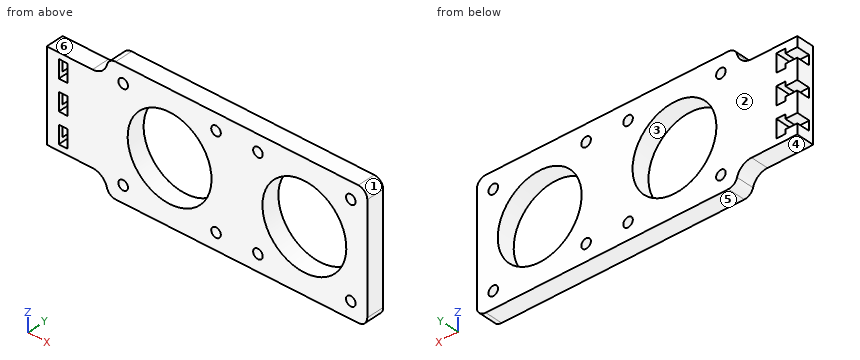
```python
from build123d import *

# Parameters (mm, degrees)
SKETCH_1_W          = 20
SKETCH_1_H          = 30
EXTRUDE_1_DEPTH     = 6
SKETCH_2_W          = 4
SKETCH_2_H          = 3.2
CUT_EXTRUDE_1_DEPTH = 4.5
SKETCH_3_W          = 3
SKETCH_3_H          = 6
CUT_EXTRUDE_2_DEPTH = 14.5
SKETCH_4_W          = 87
SKETCH_4_H          = 42
SKETCH_4_R          = 1.6
SKETCH_4_R_2        = 14
EXTRUDE_2_DEPTH     = 6
FILLET_1_R          = 3
FILLET_2_R          = 5


with BuildPart() as part:
    # 草图1 → 凸台-拉伸1 (new body)
    with BuildSketch(Plane(origin=(0, 0, 0), x_dir=(1, 0, 0), z_dir=(0, 1, 0))):
        with Locations((10, 15)):
            Rectangle(SKETCH_1_W, SKETCH_1_H)
    extrude(amount=EXTRUDE_1_DEPTH)

    # 草图2 → 切除-拉伸1 (cut)
    with BuildSketch(Plane(origin=(0, 6, 0), x_dir=(1, 0, 0), z_dir=(0, 1, 0))):
        with Locations((2, 5)):
            Rectangle(SKETCH_2_W, SKETCH_2_H)
        with Locations((2, 15)):
            Rectangle(SKETCH_2_W, SKETCH_2_H)
        with Locations((2, 25)):
            Rectangle(SKETCH_2_W, SKETCH_2_H)
    extrude(amount=-CUT_EXTRUDE_1_DEPTH, mode=Mode.SUBTRACT)

    # 草图3 → 切除-拉伸2 (cut)
    with BuildSketch(Plane(origin=(0, 6, 0), x_dir=(1, 0, 0), z_dir=(0, 1, 0))):
        with Locations((5.5, 5)):
            Rectangle(SKETCH_3_W, SKETCH_3_H)
        with Locations((5.5, 15)):
            Rectangle(SKETCH_3_W, SKETCH_3_H)
        with Locations((5.5, 25)):
            Rectangle(SKETCH_3_W, SKETCH_3_H)
    extrude(amount=-CUT_EXTRUDE_2_DEPTH, mode=Mode.SUBTRACT)

    # 草图4 → 凸台-拉伸2 (add)
    with BuildSketch(Plane.XZ):
        with Locations((63.5, -15)):
            Rectangle(SKETCH_4_W, SKETCH_4_H)
        with Locations(Location((25.5, 0.5, 0), (0, 0, 270))):
            Circle(SKETCH_4_R, mode=Mode.SUBTRACT)
        with Locations(Location((25.5, -30.5, 0), (0, 0, 90))):
            Circle(SKETCH_4_R, mode=Mode.SUBTRACT)
        with Locations(Location((56.5, -30.5, 0), (0, 0, 90))):
            Circle(SKETCH_4_R, mode=Mode.SUBTRACT)
        with Locations(Location((56.5, 0.5, 0), (0, 0, 270))):
            Circle(SKETCH_4_R, mode=Mode.SUBTRACT)
        with Locations(Location((41, -15, 0), (0, 0, 270))):
            Circle(SKETCH_4_R_2, mode=Mode.SUBTRACT)
        with Locations(Location((86, -15, 0), (0, 0, 270))):
            Circle(SKETCH_4_R_2, mode=Mode.SUBTRACT)
        with Locations(Location((70.5, 0.5, 0), (0, 0, 270))):
            Circle(SKETCH_4_R, mode=Mode.SUBTRACT)
        with Locations(Location((101.5, 0.5, 0), (0, 0, 90))):
            Circle(SKETCH_4_R, mode=Mode.SUBTRACT)
        with Locations(Location((101.5, -30.5, 0), (0, 0, 270))):
            Circle(SKETCH_4_R, mode=Mode.SUBTRACT)
        with Locations(Location((70.5, -30.5, 0), (0, 0, 90))):
            Circle(SKETCH_4_R, mode=Mode.SUBTRACT)
    extrude(amount=-EXTRUDE_2_DEPTH)

    # 圆角1
    fillet_1_edges = [part.edges().sort_by_distance(p)[0] for p in [
        (20, 3, -36),
        (107, 3, 6),
        (107, 3, -36),
        (20, 3, 6),
    ]]
    fillet(fillet_1_edges, radius=FILLET_1_R)

    # 圆角2
    fillet_2_edges = [part.edges().sort_by_distance(p)[0] for p in [
        (20, 3, -30),
        (20, 3, 0),
    ]]
    fillet(fillet_2_edges, radius=FILLET_2_R)


solid = part.part
```
Design review of the part built by this model. Coordinates are the model's own, in mm. Face numbers are marked on the shaded views. A direction names the side the tool comes from. Coordinates: 2 decimals unless noted, no trailing zeros. Order: outer loops, then holes, each group sorted by start corner. A loop starts at its lowest first (then second) coordinate and runs counter-clockwise, first axis right, second up. Notation, with made-up numbers: (52.25, 5.5) - (60.25, 5.5) arc R34 cw to (60.25, 39.5) - close; hole circle Ø6 at (17.5, 83). An arc over 180 degrees is marked (long way). Answer in a Markdown table with one row per item.
(1) Consider section B-B on x = 101.5. State the section outline as (y, z) points, plus the area to 3 significant figures.
Checked values:
| item | result |
|---|---|
| outline | (0, -36) - (6, -36) - (6, -32.1) - (0, -32.1) - close; (0, -28.9) - (6, -28.9) - (6, -1.1) - (0, -1.1) - close; (0, 2.1) - (6, 2.1) - (6, 6) - (0, 6) - close |
| area | 214 mm^2 |
(2) The part is to be moulded in two halves that separate along Z. For the marked faces 1, 2 and 3, say which applies: released by +Z, released by -Z, zero draft, split by the parting line, or undercut.
Checked values:
| item | result |
|---|---|
| face 1 | released by +Z |
| face 2 | zero draft |
| face 3 | undercut |
(3) Consider section A-A on z = -15. State the section outline as (x, y) points.
Checked values:
| item | result |
|---|---|
| outline | (0, 0) - (4, 0) - (4, 1.5) - (0, 1.5) - close; (7, 0) - (27, 0) - (27, 6) - (7, 6) - close; (55, 0) - (72, 0) - (72, 6) - (55, 6) - close; (100, 0) - (107, 0) - (107, 6) - (100, 6) - close |
(4) Consider section D-D on y = 4. Give the number of separate pieces and of enclosed holes in the cut face, plus the area to 3 significant figures.
Checked values:
| item | result |
|---|---|
| separate pieces | 1 |
| enclosed holes | 10 |
| area | 2,870 mm^2 |
(5) Consider section C-C on x = 86. State the section outline as (y, z) points, plus the area to 3 significant figures.
Checked values:
| item | result |
|---|---|
| outline | (0, -36) - (6, -36) - (6, -29) - (0, -29) - close; (0, -1) - (6, -1) - (6, 6) - (0, 6) - close |
| area | 84.0 mm^2 |
(6) Clearance check with flat-ended pins moving along their axes: pin 1 (2.5 mm diameter, centred on x = 6, y = 3, fed in from -Z); pin 2 (3.5 mm diameter, centred on x = 6, y = 4.5, fed in from +Z); pin 3 (2.5 mm diameter, centred on x = 70.5, z = 0.5, fed in from -Y). State where each tip first meets the part, or that it passes through.
Checked values:
| item | result |
|---|---|
| pin 1 | z = -30 |
| pin 2 | z = 0 |
| pin 3 | through |
(7) Wall thickness on line 1 along X through (y, z) = (3.45, -15); line 2 along Z through (x, y) = (101.5, 2.6); line 3 along X through (y, z) = (1.25, -31): over which ranges is each line inside the solid? List them lowest first. Write a range as from..to.
Checked values:
| item | result |
|---|---|
| line 1 | 7..27, 55..72, 100..107 |
| line 2 | -36..-32.1, -28.9..-1.1, 2.1..6 |
| line 3 | 18.25..23.98, 27.02..54.98, 58.02..68.98, 72.02..99.98, 103.02..107 |
(8) For the marked faces 4, 5 and 6, list the 3-axis set-ups (+Z, -Z, +X, -X, +Y, -Y) from which the entire face can be reached by the end or side of a thin tool; tool diameter is ignored.
Checked values:
| item | result |
|---|---|
| face 4 | -Z, -X, +Y, -Y |
| face 5 | -Z, +X, -X, +Y, -Y |
| face 6 | +Z, -X, +Y, -Y |
